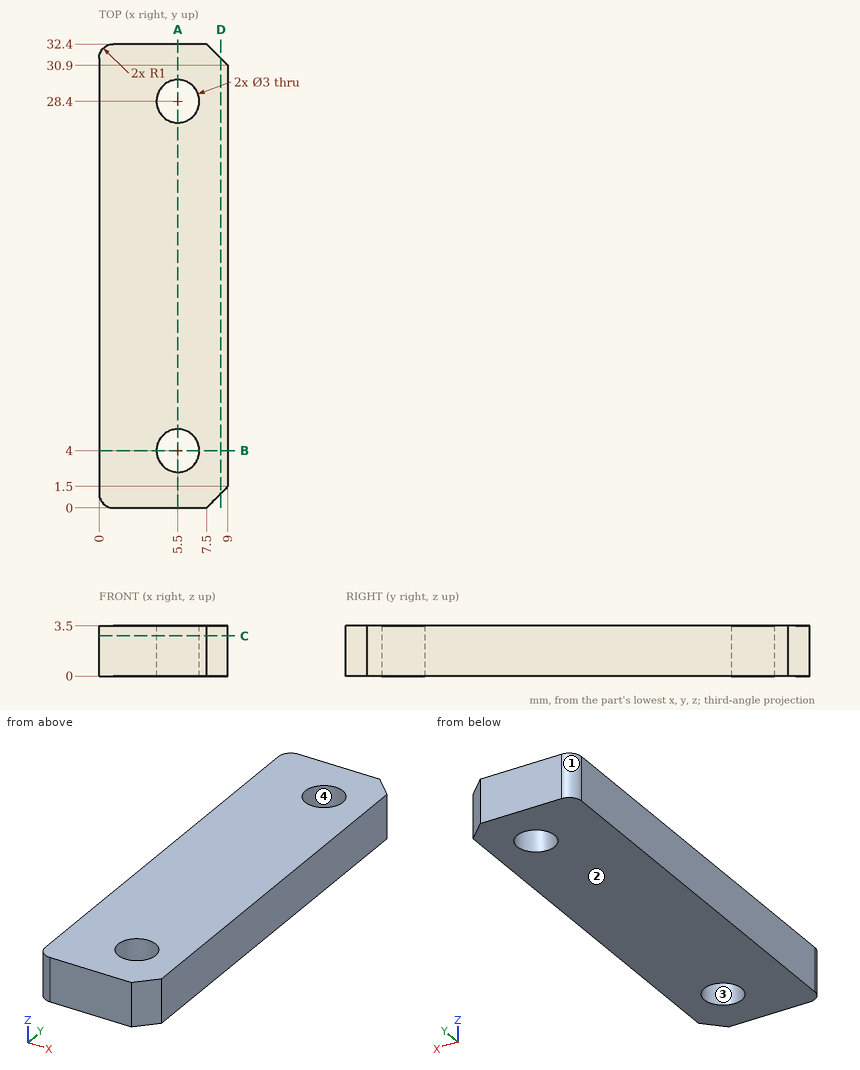
Drawing for the job (mm, zero at the part's lowest x, y, z). Coordinates: 2 decimals unless noted, no trailing zeros. Write each loop counter-clockwise with the first axis right and the second up, starting at its lowest first coordinate (ties: lowest second). Pieces come first, ordered by that corner, then holes. Notation, with made-up numbers: (-13, 24.25) -> (35, 24.25) arc R25 cw to (35, 49.25) -> close; hole circle Ø3 at (-2.75, -25). An arc over 180 degrees is marked (long way). One line per item, written item: value. Start each with the question number.
1) Slice it at B-B on y = 4. Write the cut outline in (x, z), then the cut area to 3 significant figures.
2) Slice it at D-D on x = 8.5. Write the cut outline in (y, z).
3) Slice it at C-C on z = 2.8. Write the cut outline in (x, y).
4) Flat gauge pin, fed straight in: pin 1 Ø3 at (x, y) = (2.5, 4) entering from -Z. Where does the tip first touch, or does it go through?
5) Pull direction Y, two halves, no side cores. Call the marked faces 1, 2, 3 and 4: +Y half, -Y half, draft (parallel to the pull), parting line (faces both ways), or undercut.
6) Slice it at A-A on x = 5.5. Write the cut outline in (y, z), then the cut area to 3 significant figures.
7) Probe probe 1 along Y at (x, z) = (5.5, 1.35); probe 2 along Y at (x, z) = (5, 1.95); probe 3 along X at (y, z) = (29, 0.45). List the from-to ranges inside material, lowest first.
Answers follow:
1. outline: (0, 0) -> (4, 0) -> (4, 3.5) -> (0, 3.5) -> close; (7, 0) -> (9, 0) -> (9, 3.5) -> (7, 3.5) -> close
1. area: 21.0 mm2
2. outline: (1, 0) -> (31.4, 0) -> (31.4, 3.5) -> (1, 3.5) -> close
3. outline: (0, 1) arc R1 ccw to (1, 0) -> (7.5, 0) -> (9, 1.5) -> (9, 30.9) -> (7.5, 32.4) -> (1, 32.4) arc R1 ccw to (0, 31.4) -> close; hole circle Ø3 at (5.5, 4); hole circle Ø3 at (5.5, 28.4)
4. pin 1: z = 0
5. face 1: +Y half
5. face 2: draft
5. face 3: undercut
5. face 4: undercut
6. outline: (0, 0) -> (2.5, 0) -> (2.5, 3.5) -> (0, 3.5) -> close; (5.5, 0) -> (26.9, 0) -> (26.9, 3.5) -> (5.5, 3.5) -> close; (29.9, 0) -> (32.4, 0) -> (32.4, 3.5) -> (29.9, 3.5) -> close
6. area: 92.4 mm2
7. probe 1: 0 to 2.5, 5.5 to 26.9, 29.9 to 32.4
7. probe 2: 0 to 2.59, 5.41 to 26.99, 29.81 to 32.4
7. probe 3: 0 to 4.13, 6.87 to 9
